Here's how the part is built. I have some questions about the finished solid (model axes, mm). A direction names the side the tool comes from. Coordinates: 2 decimals unless noted, no trailing zeros. Order: outer loops, then holes, each group sorted by start corner. A loop starts at its lowest first (then second) coordinate and runs counter-clockwise, first axis right, second up. Notation, with made-up numbers: (60, 27) - (66, 27) arc R7 ccw to (66, 31) - close; hole circle Ø1 at (62.5, -8). An arc over 180 degrees is marked (long way). Answer as CSV lines item,"result". Start each with the question number.
Q1. Suppose I cut it at A-A (z = -108.5). Please give me the cut outline in (x, y), then the cut area to 3 significant figures.
Q2. I need wall thicknesses on line 1 (X direction, y = 1.55, z = -146); line 2 (Z direction, x = 51.5, y = 2.45); line 3 (X direction, y = 1.3, z = -159). Which ranges of each line are inside material? Lowest first, please.
Q3. For faces 1 (the face through (69.736, 1.972, -162.92)), 2 (the face through (59.97, 3.26, -105.4)), 3 (the face through (73.296, 3, -117)), which set-ups out of +Z, -Z, +X, -X, +Y, -Y let a thin tool reach every point of the face, with its end or its side?
Q4. Suppose I cut it at C-C (z = -116.5). Please give me the cut outline in (x, y), then the cut area to 3 significant figures.
Q5. Suppose I cut it at B-B (y = 1.2). Count the separate pieces of the cut face and the enclosed holes in it, then the cut area to 3 significant figures.
Q6. Thinking about a two-plate mould opening in X: for faces 4 (the face through (94.482, 1.972, -151.586)), 5 (the face through (65.09, 1.97, -163.78)), which applies, released by +X, released by -X, zero draft, split by the parting line, or undercut?
Q7. For pin 1 Ø1.5 at (y, z) = (2, -142.5) entering from -X; pin 2 Ø11 at (x, z) = (51.56, -152.39) entering from +Y; pin 3 Ø0.8 at (y, z) = (3.5, -120) entering from -X; pin 4 Ø14.5 at (x, z) = (68, -126.5) entering from -Y, each with a flat end and sliding along its axis, tell me the tip position at first contact or that it passes through.
Autodesk Inventor part; units mm, degrees
ref_plane "YZ Plane" through (0, 0, 0) normal (1, 0, 0) x (0, 1, 0)
ref_plane "XZ Plane" through (0, 0, 0) normal (0, 1, 0) x (-1, 0, 0)
ref_plane "XY Plane" through (0, 0, 0) normal (0, 0, 1) x (1, 0, 0)
sketch "Sketch1" plane through (0, 0, 0) normal (0, 1, 0) x (-1, 0, 0)
  arc A0 (-50.2935, -141.9625) -> (-50.5085, -138.2118) centre (-57.4787, -140.493) ccw
  arc A1 (-49.4604, -134.8668) -> (-50.5085, -138.2118) centre (-45.5145, -137.94) ccw
  arc A2 (-52.2706, -141.9093) -> (-53.5294, -134.3132) centre (-66.0628, -140.2926) ccw
  arc A3 (-60.8507, -147.4866) -> (-64.2809, -146.6761) centre (-66.0428, -161.7965) ccw
  circle A4 centre (-51.5636, -152.3854) radius 9
  arc A5 (-45.2271, -160.758) -> (-42.1345, -164.9104) centre (-15.6123, -141.9291) ccw
  arc A6 (-38.966, -164.9101) -> (-37.6707, -160.6686) centre (-43.0606, -161.3412) ccw
  arc A7 (-44.5421, -165.2935) -> (-46.8275, -161.7567) centre (-172.1244, -245.2288) ccw
  arc A8 (-37.8657, -145.4277) -> (-38.2191, -140.1494) centre (-41.6996, -143.0334) ccw
  arc A9 (-45.6096, -134.3885) -> (-38.2191, -140.1494) centre (-36.6467, -130.5112) ccw
  arc A10 (-36.1368, -156.274) -> (-37.6707, -160.6686) centre (-32.4682, -160.0194) ccw
  arc A11 (-36.1368, -156.274) -> (-34.6048, -152.385) centre (-42.1305, -151.6666) ccw
  arc A12 (-41.3682, -149.8747) -> (-38.503, -148.5121) centre (-47.6774, -132.9147) ccw
  arc A13 (-41.9398, -148.1863) -> (-37.8657, -145.4277) centre (-47.8277, -135.103) ccw
  arc A14 (-34.6048, -152.385) -> (-38.503, -148.5121) centre (-40.8573, -154.78) ccw
  arc A15 (-63.8657, -139.5775) -> (-58.174, -134.8668) centre (-65.1246, -132.2626) ccw
  arc A16 (-53.5294, -134.3132) -> (-58.174, -134.8668) centre (-55.4761, -137.7415) ccw
  arc A17 (-45.6096, -134.3885) -> (-49.4604, -134.8668) centre (-47.2959, -136.5525) ccw
  line L0 (-46.3394, -171.0352) -> (-46.3407, -171.0345)
  arc A18 (-48.8902, -170.6862) -> (-44.9412, -169.507) centre (-47.5666, -167.9168) ccw
  arc A19 (-65.6657, -161.3497) -> (-62.9245, -164.9101) centre (-62.7518, -161.9418) ccw
  arc A20 (-62.9245, -164.9101) -> (-58.2423, -160.4876) centre (-68.2851, -154.5449) ccw
  arc A21 (-56.5584, -161.6213) -> (-58.6246, -165.2834) centre (21.5695, -208.1162) ccw
  arc A22 (-58.6246, -165.2834) -> (-59.26, -166.6979) centre (-55.3426, -167.6077) ccw
  arc A23 (-59.26, -166.6979) -> (-53.816, -170.3276) centre (-55.8552, -167.4887) ccw
  arc A24 (-48.8902, -170.6862) -> (-53.816, -170.3276) centre (-51.7693, -176.2225) ccw
  arc A25 (-65.6657, -161.3497) -> (-67.4979, -155.3741) centre (-72.0774, -160.047) ccw
  arc A26 (-61.8781, -150.4206) -> (-66.2243, -148.9882) centre (-82.2432, -204.906) ccw
  arc A27 (-42.1345, -164.9104) -> (-38.966, -164.9101) centre (-40.5505, -161.8463) ccw
  arc A28 (-44.9412, -169.507) -> (-44.5421, -165.2935) centre (-48.2055, -167.0721) ccw
  arc A29 (-76.2935, -141.9625) -> (-76.5085, -138.2118) centre (-83.4787, -140.493) ccw
  arc A30 (-75.4604, -134.8668) -> (-76.5085, -138.2118) centre (-71.5145, -137.94) ccw
  arc A31 (-78.2706, -141.9093) -> (-79.5294, -134.3132) centre (-92.0628, -140.2926) ccw
  arc A32 (-86.8507, -147.4866) -> (-90.2809, -146.6761) centre (-92.0428, -161.7965) ccw
  circle A33 centre (-77.5636, -152.3854) radius 9
  arc A34 (-71.2271, -160.758) -> (-68.1345, -164.9104) centre (-41.6123, -141.9291) ccw
  arc A35 (-70.5421, -165.2935) -> (-72.8275, -161.7567) centre (-198.1244, -245.2288) ccw
  arc A36 (-63.8657, -145.4277) -> (-64.2191, -140.1494) centre (-67.6996, -143.0334) ccw
  arc A37 (-71.6096, -134.3885) -> (-64.2191, -140.1494) centre (-62.6467, -130.5112) ccw
  arc A38 (-67.9398, -148.1863) -> (-63.8657, -145.4277) centre (-73.8277, -135.103) ccw
  arc A39 (-90.7671, -139.6764) -> (-84.174, -134.8668) centre (-91.1246, -132.2626) ccw
  arc A40 (-79.5294, -134.3132) -> (-84.174, -134.8668) centre (-81.4761, -137.7415) ccw
  arc A41 (-71.6096, -134.3885) -> (-75.4604, -134.8668) centre (-73.2959, -136.5525) ccw
  line L1 (-72.3394, -171.0352) -> (-72.3407, -171.0345)
  arc A42 (-74.8902, -170.6862) -> (-70.9412, -169.507) centre (-73.5666, -167.9168) ccw
  arc A43 (-91.6657, -161.3497) -> (-88.9245, -164.9101) centre (-88.7518, -161.9418) ccw
  arc A44 (-88.9245, -164.9101) -> (-84.2423, -160.4876) centre (-94.2851, -154.5449) ccw
  arc A45 (-82.5584, -161.6213) -> (-84.6246, -165.2834) centre (-4.4305, -208.1162) ccw
  arc A46 (-84.6246, -165.2834) -> (-85.26, -166.6979) centre (-81.3426, -167.6077) ccw
  arc A47 (-85.26, -166.6979) -> (-79.816, -170.3276) centre (-81.8552, -167.4887) ccw
  arc A48 (-74.8902, -170.6862) -> (-79.816, -170.3276) centre (-77.7693, -176.2225) ccw
  arc A49 (-91.6639, -144.9966) -> (-90.2809, -146.6761) centre (-87.4857, -142.9652) ccw
  arc A50 (-90.7671, -139.6764) -> (-91.6639, -144.9966) centre (-87.4857, -142.9652) ccw
  arc A51 (-91.6657, -161.3497) -> (-94.028, -154.908) centre (-98.0774, -160.047) ccw
  arc A52 (-92.2243, -148.9882) -> (-94.028, -154.908) centre (-90.5316, -152.7386) ccw
  arc A53 (-87.8781, -150.4206) -> (-92.2243, -148.9882) centre (-108.2432, -204.906) ccw
  arc A54 (-68.1345, -164.9104) -> (-64.966, -164.9101) centre (-66.5505, -161.8463) ccw
  arc A55 (-70.9412, -169.507) -> (-70.5421, -165.2935) centre (-74.2055, -167.0721) ccw
  arc A56 (-66.2243, -148.9882) -> (-67.3918, -149.7806) centre (-64.5316, -152.7386) ccw
  circle A57 centre (-51.5636, -152.3854) radius 10.5
  circle A58 centre (-77.5636, -152.3854) radius 10.5
  arc A59 (-66.5505, -161.8463) -> (-64.966, -164.9101) centre (-62.3299, -161.6052) ccw
  arc A60 (-66.5505, -161.8463) -> (-67.9398, -156.5846) centre (-74.2403, -161.0624) ccw
  arc A61 (-64.2809, -146.6761) -> (-63.8657, -139.5775) centre (-67.8597, -142.9054) ccw
  line L2 (-53.5294, -134.3132) -> (-53.5294, -99.3132)
  line L3 (-53.5294, -99.3132) -> (-75.4604, -134.8668)
  line L4 (-75.4604, -134.8668) -> (-75.4604, -99.3132)
  line L5 (-75.4604, -99.3132) -> (-53.5294, -134.3132)
  point P0 (0, 0)
  point P1 (-51.4803, -152.4063)
  point P2 (-45.3977, -162.821)
  point P3 (-45.3977, -141.9574)
  point P4 (-33.5868, -132.2626)
  point P5 (-34.505, -161.7965)
  point P6 (-36.7472, -154.5449)
  point P7 (-47.2742, -170.9723)
  point P8 (-57.8397, -162.8189)
  point P9 (-56.1478, -170.9718)
  point P10 (-71.3977, -162.821)
  point P11 (-71.3977, -141.9574)
  point P12 (-59.5868, -132.2626)
  point P13 (-60.505, -161.7965)
  point P14 (-62.7472, -154.5449)
  point P15 (-73.2742, -170.9723)
  point P16 (-83.8397, -162.8189)
  point P17 (-82.1478, -170.9718)
  dimension "d2" = 21
  dimension "d3" = 21
  dimension "d0" = 18
  dimension "d1" = 18
  dimension "d6" = 35
extrude "Extrusion1" add sketch "Sketch1" along normal blind 4 contours A0 A1 A17 A9 A8 A13 A57 | A57 | A57 A3 A61 A15 A16 A2 | A12 A14 A11 A10 A6 A27 A5 A57 | A57 A20 A19 A25 A58 A56 A26 | A41 A37 A36 A38 A58 A29 A30 | A7 A28 A18 A24 A23 A22 A21 A57 | A58 | A58 A32 A49 A50 A39 A40 A31 | A60 A59 A54 A34 A58 | A58 A44 A43 A51 A52 A53 | A35 A55 A42 A48 A47 A46 A45 A58
sketch "Sketch3" plane through (0, 4, 0) normal (0, 1, 0) x (1, 0, 0)
  arc A0 (53.5294, 134.3132) -> (58.174, 134.8668) centre (55.4761, 137.7415) ccw
  line L0 (55.4761, 133.799) -> (55.4761, 98.799)
  arc A1 (71.6096, 134.3885) -> (75.4604, 134.8668) centre (73.2959, 136.5525) ccw
  line L1 (73.2959, 133.8091) -> (73.2959, 98.8091)
  line L2 (55.4761, 133.799) -> (61.5958, 151.1662)
  line L3 (61.5958, 151.1662) -> (68.0809, 150.5767)
  line L4 (68.0809, 150.5767) -> (73.2959, 133.8091)
  line L5 (55.4761, 98.799) -> (64.5905, 112.1825)
  line L6 (64.5905, 112.1825) -> (73.2959, 98.8091)
  point P0 (0, 0)
  dimension "d7" = 35
  dimension "d8" = 35
extrude "Extrusion2" add sketch "Sketch3" against normal blind 1.5
properties part number "RosaV2"
Here are the results:
1,outline,"(55.48, 2.5) - (62.08, 2.5) - (62.08, 4) - (55.48, 4) - close; (66.99, 2.5) - (73.3, 2.5) - (73.3, 4) - (66.99, 4) - close"
1,area,"19.4 mm²"
2,line 1,"x = 38.5 to 45.22, 57.91 to 63.68, 64.5 to 71.22, 83.91 to 91"
2,line 2,"z = -169.99 to -161.39, -143.39 to -141.89"
2,line 3,"x = 37.61 to 45.46, 57.67 to 65.62, 66.79 to 71.46, 83.67 to 91.62"
3,face 1,"+Y, -Y"
3,face 2,"+Z, +Y, -Y"
3,face 3,"+Z, +X, +Y, -Y"
4,outline,"(55.48, 2.5) - (73.3, 2.5) - (73.3, 4) - (55.48, 4) - close"
4,area,"26.7 mm²"
5,separate pieces,"1"
5,enclosed holes,"2"
5,area,"1,100 mm²"
6,face 4,"released by +X"
6,face 5,"undercut"
7,pin 1,"stops at x = 37.18"
7,pin 2,"passes through"
7,pin 3,"stops at x = 55.48"
7,pin 4,"stops at y = 2.5"
